Input: part model. Units: mm. Frame: model coordinates. A direction names the side the tool comes from. Coordinates: 2 decimals unless noted, no trailing zeros. Write each loop counter-clockwise with the first axis right and the second up, starting at its lowest first coordinate (ties: lowest second). Pieces come first, ordered by that corner, then holes. Notation, with made-up numbers: (-32.75, -0.5) - (3.25, -0.5) arc R29 cw to (3.25, 32.5) - close; hole circle Ø6 at (89, -0.75). An arc over 180 degrees is marked (long way). Use CSV: the item, a comma, the result in double quotes.
```python
from build123d import *

# Parameters (mm, degrees)
SKETCH1_R               = 80
BOSS_EXTRUDE1_DEPTH     = 10
CUT_EXTRUDE1_REACH      = 115.578
SKETCH2_R               = 2.5
CUT_EXTRUDE2_REACH      = 115.578
SKETCH3_W               = 40
SKETCH3_H               = 40
CUT_EXTRUDE3_REACH      = 115.578
SKETCH5_W               = 8
SKETCH5_H               = 40
BOSS_EXTRUDE2_DEPTH     = 15
FILLET1_SIZE            = 5
CUT_EXTRUDE4_REACH      = 138.708
SKETCH6_R               = 3
FILLET1_OF_MIRROR1_SIZE = 5


with BuildPart() as part:
    # Sketch1 → Boss-Extrude1 (new body)
    with BuildSketch(Plane(origin=(0, 0, 0), x_dir=(1, 0, 0), z_dir=(0, 1, 0))):
        with Locations(Location((0, 0, 0), (0, 0, 270))):
            Circle(SKETCH1_R)
    extrude(amount=BOSS_EXTRUDE1_DEPTH)

    # Sketch2 → Cut-Extrude1 (cut, up to next)
    with BuildSketch(Plane(origin=(0, 10, 0), x_dir=(1, 0, 0), z_dir=(0, 1, 0)), mode=Mode.PRIVATE) as cut_extrude1_sk1:
        with Locations(Location((-75, 0, 0), (0, 0, 270))):
            Circle(SKETCH2_R)
    cut_extrude1_tool1 = extrude(cut_extrude1_sk1.sketch, amount=-CUT_EXTRUDE1_REACH, mode=Mode.PRIVATE) & part.part
    # Sketch2 → Cut-Extrude1 (cut, up to next)
    with BuildSketch(Plane(origin=(0, 10, 0), x_dir=(1, 0, 0), z_dir=(0, 1, 0)), mode=Mode.PRIVATE) as cut_extrude1_sk2:
        with Locations(Location((0, 75, 0), (0, 0, 270))):
            Circle(SKETCH2_R)
    cut_extrude1_tool2 = extrude(cut_extrude1_sk2.sketch, amount=-CUT_EXTRUDE1_REACH, mode=Mode.PRIVATE) & part.part
    # Sketch2 → Cut-Extrude1 (cut, up to next)
    with BuildSketch(Plane(origin=(0, 10, 0), x_dir=(1, 0, 0), z_dir=(0, 1, 0)), mode=Mode.PRIVATE) as cut_extrude1_sk3:
        with Locations(Location((75, 0, 0), (0, 0, 270))):
            Circle(SKETCH2_R)
    cut_extrude1_tool3 = extrude(cut_extrude1_sk3.sketch, amount=-CUT_EXTRUDE1_REACH, mode=Mode.PRIVATE) & part.part
    # Sketch2 → Cut-Extrude1 (cut, up to next)
    with BuildSketch(Plane(origin=(0, 10, 0), x_dir=(1, 0, 0), z_dir=(0, 1, 0)), mode=Mode.PRIVATE) as cut_extrude1_sk4:
        with Locations(Location((0, -75, 0), (0, 0, 270))):
            Circle(SKETCH2_R)
    cut_extrude1_tool4 = extrude(cut_extrude1_sk4.sketch, amount=-CUT_EXTRUDE1_REACH, mode=Mode.PRIVATE) & part.part
    add(cut_extrude1_tool1.solids().sort_by_distance((-75, 10, 0))[0], mode=Mode.SUBTRACT)
    add(cut_extrude1_tool2.solids().sort_by_distance((0, 10, -75))[0], mode=Mode.SUBTRACT)
    add(cut_extrude1_tool3.solids().sort_by_distance((75, 10, 0))[0], mode=Mode.SUBTRACT)
    add(cut_extrude1_tool4.solids().sort_by_distance((0, 10, 75))[0], mode=Mode.SUBTRACT)

    # Sketch3 → Cut-Extrude2 (cut, up to next)
    with BuildSketch(Plane(origin=(0, 10, 0), x_dir=(1, 0, 0), z_dir=(0, 1, 0)), mode=Mode.PRIVATE) as cut_extrude2_sk1:
        Rectangle(SKETCH3_W, SKETCH3_H)
    cut_extrude2_tool1 = extrude(cut_extrude2_sk1.sketch, amount=-CUT_EXTRUDE2_REACH, mode=Mode.PRIVATE) & part.part
    add(cut_extrude2_tool1.solids().sort_by_distance((0, 10, 0))[0], mode=Mode.SUBTRACT)

    # Sketch4 → Cut-Extrude3 (cut, up to next)
    with BuildSketch(Plane(origin=(0, 10, 0), x_dir=(1, 0, 0), z_dir=(0, 1, 0)), mode=Mode.PRIVATE) as cut_extrude3_sk1:
        with BuildLine():
            Line((23.5, -45), (-18.5, -45))
            Line((-18.5, -45), (-18.5, -46.75))
            Line((-18.5, -46.75), (-23, -46.75))
            ThreePointArc((-23, -46.75), (-25.25, -49), (-23, -51.25))
            Line((-23, -51.25), (-18.5, -51.25))
            Line((-18.5, -51.25), (-18.5, -56.75))
            Line((-18.5, -56.75), (-23, -56.75))
            ThreePointArc((-23, -56.75), (-25.25, -59), (-23, -61.25))
            Line((-23, -61.25), (-18.5, -61.25))
            Line((-18.5, -61.25), (-18.5, -63))
            Line((-18.5, -63), (23.5, -63))
            Line((23.5, -63), (23.5, -61.25))
            Line((23.5, -61.25), (28, -61.25))
            ThreePointArc((28, -61.25), (30.25, -59), (28, -56.75))
            Line((28, -56.75), (23.5, -56.75))
            Line((23.5, -56.75), (23.5, -51.25))
            Line((23.5, -51.25), (28, -51.25))
            ThreePointArc((28, -51.25), (30.25, -49), (28, -46.75))
            Line((28, -46.75), (23.5, -46.75))
            Line((23.5, -46.75), (23.5, -45))
        make_face()
    cut_extrude3_tool1 = extrude(cut_extrude3_sk1.sketch, amount=-CUT_EXTRUDE3_REACH, mode=Mode.PRIVATE) & part.part
    add(cut_extrude3_tool1.solids().sort_by_distance((2.5, 10, 54))[0], mode=Mode.SUBTRACT)

    # Sketch5 → Boss-Extrude2 (add)
    with BuildSketch(Plane(origin=(0, 10, 0), x_dir=(1, 0, 0), z_dir=(0, 1, 0))):
        with Locations((-24, 0)):
            Rectangle(SKETCH5_W, SKETCH5_H)
    boss_extrude2 = extrude(amount=BOSS_EXTRUDE2_DEPTH)

    # Fillet1
    fillet1_edges = [part.edges().sort_by_distance(p)[0] for p in [
        (-24, 25, -20),
        (-24, 25, 20),
    ]]
    chamfer(fillet1_edges, length=FILLET1_SIZE)

    # Sketch6 → Cut-Extrude4 (cut, up to next)
    with BuildSketch(Plane.ZY.offset(28), mode=Mode.PRIVATE) as cut_extrude4_sk1:
        with Locations((0, 17.5)):
            Circle(SKETCH6_R)
    cut_extrude4_tool1 = extrude(cut_extrude4_sk1.sketch, amount=-CUT_EXTRUDE4_REACH, mode=Mode.PRIVATE) & part.part
    cut_extrude4 = cut_extrude4_tool1.solids().sort_by_distance((-28, 17.5, 0))[0]
    add(cut_extrude4, mode=Mode.SUBTRACT)

    # Mirror1: Boss-Extrude2, Cut-Extrude4 across plane
    add(boss_extrude2.mirror(Plane.ZY))
    add(cut_extrude4.mirror(Plane.ZY), mode=Mode.SUBTRACT)

    # Fillet1 of Mirror1
    fillet1_of_mirror1_edges = [part.edges().sort_by_distance(p)[0] for p in [
        (24, 25, -20),
        (24, 25, 20),
    ]]
    chamfer(fillet1_of_mirror1_edges, length=FILLET1_OF_MIRROR1_SIZE)


solid = part.part
```
(1) Cut plane B-B on x = 0. Return loops of the section in (y, z), and give its area (3 significant figures).
Check values:
outline,"(0, -80) - (10, -80) - (10, -77.5) - (0, -77.5) - close; (0, -72.5) - (10, -72.5) - (10, -20) - (0, -20) - close; (0, 20) - (10, 20) - (10, 45) - (0, 45) - close; (0, 63) - (10, 63) - (10, 72.5) - (0, 72.5) - close; (0, 77.5) - (10, 77.5) - (10, 80) - (0, 80) - close"
area,"920 mm^2"
(2) Draft query along Z for faces 5 (the flat face through (-18.5, 5, 54)), 6 (the flat face through (-24, 15, 20)), 7 (the flat face through (-28, 14, 0)), 8 (the flat face through (-21, 5, 61.25)). Return one class per face: pulls with the +Z half, pulls with the -Z half, needs draft (parallel to the pull), parting line crosses it, or undercut.
Check values:
face 5,"undercut"
face 6,"pulls with the +Z half"
face 7,"needs draft"
face 8,"undercut"
(3) Reachability of faces 1 (the flat face through (28, 14, 0)), 2 (the cylindrical face through (24.06, 14.57, -0.65)), 3 (the cylindrical face through (-25.25, 5.07, 58.95)), 4 (the flat face through (24, 15, 20)) from +Z, -Z, +X, -X, +Y, -Y: full face, straight path, thin tool, end or side. Return the list, or none.
Check values:
face 1,"+Z, -Z, +X, +Y"
face 2,"+X, -X"
face 3,"+Y, -Y"
face 4,"+Z, +X, -X, +Y"
(4) Cut plane D-D on y = 7.5. State how many separate pieces and enclosed holes the cut face has, and give its area (3 significant figures).
Check values:
separate pieces,"1"
enclosed holes,"6"
area,"17,600 mm^2"
(5) Cut plane A-A on y = 17.5. Return loops of the section in (x, z), and give its area (3 significant figures).
Check values:
outline,"(-28, -20) - (-20, -20) - (-20, -3) - (-28, -3) - close; (-28, 3) - (-20, 3) - (-20, 20) - (-28, 20) - close; (20, -20) - (28, -20) - (28, -3) - (20, -3) - close; (20, 3) - (28, 3) - (28, 20) - (20, 20) - close"
area,"544 mm^2"
(6) Pin query (flat end, axial travel): pin 1 Ø6 at (y, z) = (5, 54) entering from -X; pin 2 Ø5 at (x, z) = (-46.5, -53) entering from +Y; pin 3 Ø2 at (y, z) = (7.5, 43.5) entering from -X; pin 4 Ø3 at (x, z) = (-75, 0) entering from -Y. Return the tip coordinate at first contact, or that it passes through.
Check values:
pin 1,"x = -61.64"
pin 2,"y = 10"
pin 3,"x = -67.78"
pin 4,"through"
(7) Cut plane C-C on z = 0. Return loops of the section in (x, y), and give its area (3 significant figures).
Check values:
outline,"(-80, 0) - (-77.5, 0) - (-77.5, 10) - (-80, 10) - close; (-72.5, 0) - (-20, 0) - (-20, 14.5) - (-28, 14.5) - (-28, 10) - (-72.5, 10) - close; (-28, 20.5) - (-20, 20.5) - (-20, 25) - (-28, 25) - close; (20, 0) - (72.5, 0) - (72.5, 10) - (28, 10) - (28, 14.5) - (20, 14.5) - close; (20, 20.5) - (28, 20.5) - (28, 25) - (20, 25) - close; (77.5, 0) - (80, 0) - (80, 10) - (77.5, 10) - close"
area,"1,240 mm^2"
(8) Ray query, probe 1 along Y at (x, z) = (23, 0); probe 2 along X at (y, z) = (19, -17); probe 3 along Z at (x, y) = (27.5, 4.25). Return the intervals inside material, ascending. Write a range as from..to.
Check values:
probe 1,"0..14.5, 20.5..25"
probe 2,"-28..-20, 20..28"
probe 3,"-75.12..46.75, 51.25..56.75, 61.25..75.12"
